Source: CAD feature listing. Evaluate the final solid. Frame: model axes, mm. A direction names the side the tool comes from. Coordinates: 2 decimals unless noted, no trailing zeros. Loops run counter-clockwise (first coordinate to the right, second up) from the corner with the lowest first, then second, coordinate; pieces in that order, holes last. Notation, with made-up numbers: (-22.75, -3) - (-12.75, -3) arc R21 ccw to (-12.75, 32) - close; hole circle Ø4 at (36.25, 17). An arc over 180 degrees is marked (long way). Use one line per item in the form item = value. Start each with the question number.
Solid Edge part; units mm, degrees
sketch "Sketch1" plane through (0, 0, 0) normal (0, -1, 0) x (1, 0, 0)
  line L0 (-2.5, -2.25) -> (2.5, -2.25)
  line L1 (2.5, -2.25) -> (2.5, 2.25)
  line L2 (2.5, 2.25) -> (-2.5, 2.25)
  line L3 (-2.5, 2.25) -> (-2.5, -2.25)
  dimension "D1" = 2.5
  dimension "D2" = 2.5
extrude "Protrusion1" add sketch "Sketch1" along normal mid plane 36
fillet "Round_2" radius 1 3 edges at (0, 18, 2.25) (-2.5, 18, 0) (0, 18, -2.25)
mirror "Mirror1" about plane through (0, 0, 0) normal (0, -1, 0) of "Round_2"
sketch "Sketch2" plane through (-2.5, 0, 0) normal (-1, 0, 0) x (0, -1, 0)
  line L0 (7.5, -2.25) -> (-7.5, -2.25)
  line L1 (-7.5, -2.25) -> (-7.5, 2.25)
  line L2 (-7.5, 2.25) -> (7.5, 2.25)
  line L3 (7.5, 2.25) -> (7.5, -2.25)
  dimension "D1" = 7.5
extrude "ExtrudedProtrusion_2" add sketch "Sketch2" along normal blind 25
sketch "Sketch3" plane through (0, 0, 0) normal (0, 0, 1) x (1, 0, 0)
  line L0 (-21.5, -7.5) -> (-27.5, -7.5)
  line L1 (-27.5, -7.5) -> (-27.5, 7.5)
  line L2 (-27.5, 7.5) -> (-21.5, 7.5)
  line L3 (-21.5, 7.5) -> (-21.5, -7.5)
  dimension "D1" = 27.5
extrude "ExtrudedProtrusion_3" add sketch "Sketch3" along normal mid plane 15
fillet "Round_3" radius 5 2 edges at (-21.5, 0, 2.25) (-21.5, 0, -2.25)
fillet "Round_4" radius 1 4 edges at (-24.5, -7.5, 7.5) (-24.5, 7.5, 7.5) (-24.5, -7.5, -7.5) (-24.5, 7.5, -7.5)
fillet "Round_5" radius 3 2 edges at (-2.5, -7.5, 0) (-2.5, 7.5, 0)
(1) Contact query for flat-ended pins moving along their axis: pin 1 (3 mm diameter, centred on x = -7.5, z = -0.5, fed in from -Y); pin 2 (2 mm diameter, centred on y = 12.5, z = 0, fed in from -X); pin 3 (2 mm diameter, centred on y = 7, z = -2.5, fed in from +X); pin 4 (3 mm diameter, centred on x = -21.5, y = -9.5, fed in from +Z). Output: stop coordinate, or through.
(2) Material intervals for line 1 (Z direction, x = -10, y = 6); line 2 (X direction, y = -11.5, z = 1.5); line 3 (Y direction, x = -25.5, z = -3.25), sorted ascending.
(3) Cut plane A-A, the plane x = 0.5. Output: boundary loops of the cut face in (y, z), plus the area to 3 significant figures.
(4) Cut plane B-B, the plane y = -1. Output: boundary loops of the cut face in (x, z).
(5) Access query for faces 1 (the face through (-19, -7.5, 0)), 2 (the face through (-2.5, 14, 0)), 3 (the face through (-5, 0, 2.25)). Directions: +Z, -Z, +X, -X, +Y, -Y. A direction counts if a zero-diameter tool reaches every point of the face in a straight line with its end or side. Return the directions, or none.
(6) Cut plane D-D, the plane x = -23. Output: boundary loops of the cut face in (y, z), plus the area to 3 significant figures.
(7) Cut plane C-C, the plane z = -4.25. Output: boundary loops of the cut face in (x, y).
Recorded:
q1.pin_1 = -7.5
q1.pin_2 = -2.5
q1.pin_3 = 2.5
q1.pin_4 = through
q2.line_1 = -2.25 to 2.25
q2.line_2 = -2.5 to 2.5
q2.line_3 = -7.5 to 7.5
q3.outline = (-18, -1.25) arc R1 ccw to (-17, -2.25) - (17, -2.25) arc R1 ccw to (18, -1.25) - (18, 1.25) arc R1 ccw to (17, 2.25) - (-17, 2.25) arc R1 ccw to (-18, 1.25) - close
q3.area = 161 mm²
q4.outline = (-27.5, -7.5) - (-21.5, -7.5) - (-21.5, -7.25) arc R5 cw to (-16.5, -2.25) - (2.5, -2.25) - (2.5, 2.25) - (-16.5, 2.25) arc R5 cw to (-21.5, 7.25) - (-21.5, 7.5) - (-27.5, 7.5) - close
q5.face_1 = +Z, -Z, -X, -Y
q5.face_2 = +Z, -Z, -X, +Y
q5.face_3 = +Z, +X, +Y, -Y
q6.outline = (-7.5, -6.5) arc R1 ccw to (-6.5, -7.5) - (6.5, -7.5) arc R1 ccw to (7.5, -6.5) - (7.5, 6.5) arc R1 ccw to (6.5, 7.5) - (-6.5, 7.5) arc R1 ccw to (-7.5, 6.5) - close
q6.area = 224 mm²
q7.outline = (-27.5, -7.5) - (-20.5, -7.5) - (-20.5, 7.5) - (-27.5, 7.5) - close
